Verification items for the finished model (mm, model axes). Face numbers are marked on the shaded views. A direction names the side the tool comes from. Give positions to 0.01 mm unless a question says otherwise; leave off trailing zeros. Loops run counter-clockwise (first coordinate to the right, second up) from the corner with the lowest first, then second, coordinate; pieces in that order, holes last. Notation, with made-up numbers: (9, 32) - (27, 32) arc R7 ccw to (27, 43) - close; hole circle Ø6 at (12.25, 68). An arc over 180 degrees is marked (long way). One line per question, with ' | ' between items. Start each with the question number.
1. Section check B-B, the plane x = -20. Enter the section's corners in (y, z), then the cut area to 3 significant figures.
2. Tool access check on the marked faces 1 and 2. Record the directions out of +Z, -Z, +X, -X, +Y, -Y that give a thin tool (end or side, any length) a straight path to the whole face; none if there is none.
3. Thickness scan on line 1 along Z through (x, y) = (-20, -6); line 2 along X through (y, z) = (-6.5, 4); line 3 along Z through (x, y) = (15.5, -12.75). Record the ranges inside material, lowest first. Write a range as from..to.
4. Section check A-A, the plane y = -13. Enter the section's corners in (x, z), then the cut area to 3 significant figures.
5. Depth check by flat-ended pin: pin 1 Ø7.5 at (y, z) = (-18.5, -13.5) entering from -X; pin 2 Ø7.5 at (x, y) = (-13.5, -13.5) entering from -Z. Enter the tip coordinate at first touch or a pass-through.
6. Section check C-C, the plane z = -5. Enter the section's corners in (x, y).
from build123d import *

# Parameters (mm, degrees)
F4_W     = 50
F4_H     = 65
F0_DEPTH = 25
F1_W     = 30
F1_H     = 30
F2_DEPTH = 25
F3_SIZE  = 5


with BuildPart() as f0:
    # F4 (on Front) → F0 (new body)
    with BuildSketch(Plane.XZ):
        with Locations((-5, 7.461506)):
            Rectangle(F4_W, F4_H)
    extrude(amount=F0_DEPTH)

    # F1 (on face) → F2 (cut)
    with BuildSketch(Plane.XZ.offset(25)):
        with Locations((-15, -10.038494)):
            Rectangle(F1_W, F1_H)
    extrude(amount=-F2_DEPTH, mode=Mode.SUBTRACT)

    # F3
    f3_edges = [f0.edges().sort_by_distance(p)[0] for p in [
        (20, -12.5, 39.961506),
    ]]
    chamfer(f3_edges, length=F3_SIZE)


solid = f0.part
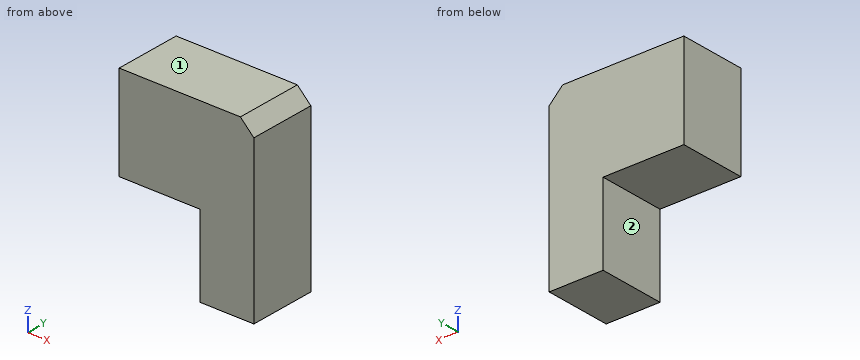
Results list:
1) outline: (-25, 4.96) - (0, 4.96) - (0, 39.96) - (-25, 39.96) - close | area: 875 mm²
2) face 1: +Z, +X, -X, +Y, -Y | face 2: -Z, -X, +Y, -Y
3) line 1: 4.96..39.96 | line 2: 0..20 | line 3: -25.04..39.46
4) outline: (-30, 4.96) - (0, 4.96) - (0, -25.04) - (20, -25.04) - (20, 34.96) - (15, 39.96) - (-30, 39.96) - close | area: 2,340 mm²
5) pin 1: x = 0 | pin 2: z = 4.96
6) outline: (0, -25) - (20, -25) - (20, 0) - (0, 0) - close
